```python
from build123d import *

# Parameters (mm, degrees)
F0_R     = 4.5
F0_W     = 85
F0_H     = 160
F0_H_2   = 10
F0_R_2   = 2
F1_DEPTH = 30
F2_W     = 85
F2_H     = 40
F2_R     = 4.5
F2_H_2   = 5
F3_DEPTH = 5
F4_W     = 85
F4_H     = 45
F4_R     = 2
F4_R_2   = 6
F5_DEPTH = 15
F4_R_3   = 4.5
F6_DEPTH = 15
F7_DEPTH = 25


with BuildPart() as f1:
    # F0 (on Top) → F1 (new body)
    with BuildSketch(Plane.XY):
        Polygon((115, -285), (115, 205), (265, 205), (265, 235), (-180, 235), (-180, 205), (-30, 205), (-30, -285), (-180, -285), (-180, -315), (265, -315), (265, -285), align=None)
        with Locations((-165, -300)):
            Circle(F0_R, mode=Mode.SUBTRACT)
        with Locations((250, -300)):
            Circle(F0_R, mode=Mode.SUBTRACT)
        Polygon((0, -120), (0, 0), (85, 0), (85, -120), (85, -130), (85, -285), (0, -285), (0, -130), align=None, mode=Mode.SUBTRACT)
        with Locations((27.5, 10)):
            Circle(F0_R, mode=Mode.SUBTRACT)
        with Locations((27.5, 29)):
            Circle(F0_R, mode=Mode.SUBTRACT)
        with Locations((-165, 220)):
            Circle(F0_R, mode=Mode.SUBTRACT)
        with Locations((57.5, 10)):
            Circle(F0_R, mode=Mode.SUBTRACT)
        with Locations((57.5, 29)):
            Circle(F0_R, mode=Mode.SUBTRACT)
        with Locations((42.5, 125)):
            Rectangle(F0_W, F0_H, mode=Mode.SUBTRACT)
        with Locations((250, 220)):
            Circle(F0_R, mode=Mode.SUBTRACT)
        with Locations((42.5, -125)):
            Rectangle(F0_W, F0_H_2)
        with Locations((10, -125)):
            Circle(F0_R_2, mode=Mode.SUBTRACT)
        with Locations((75, -125)):
            Circle(F0_R_2, mode=Mode.SUBTRACT)
    extrude(amount=F1_DEPTH)

    # F2 (on face) → F3 (cut)
    with BuildSketch(Plane.XY.offset(30)):
        with Locations((42.5, 20)):
            Rectangle(F2_W, F2_H)
        with Locations((27.5, 10)):
            Circle(F2_R, mode=Mode.SUBTRACT)
        with Locations((27.5, 29)):
            Circle(F2_R, mode=Mode.SUBTRACT)
        with Locations((57.5, 10)):
            Circle(F2_R, mode=Mode.SUBTRACT)
        with Locations((57.5, 29)):
            Circle(F2_R, mode=Mode.SUBTRACT)
        with Locations((42.5, 42.5)):
            Rectangle(F2_W, F2_H_2)
    extrude(amount=-F3_DEPTH, mode=Mode.SUBTRACT)

    # F4 (on face) + F0 (on Top) → F5 (cut)
    with BuildSketch(Plane.XY):
        with Locations((42.5, 22.5)):
            Rectangle(F4_W, F4_H)
        with Locations((10, 5)):
            Circle(F4_R, mode=Mode.SUBTRACT)
        with Locations((27.5, 10)):
            Circle(F4_R_2, mode=Mode.SUBTRACT)
        with Locations((10, 40)):
            Circle(F4_R, mode=Mode.SUBTRACT)
        with Locations((27.5, 29)):
            Circle(F4_R_2, mode=Mode.SUBTRACT)
        with Locations((57.5, 10)):
            Circle(F4_R_2, mode=Mode.SUBTRACT)
        with Locations((75, 5)):
            Circle(F4_R, mode=Mode.SUBTRACT)
        with Locations((57.5, 29)):
            Circle(F4_R_2, mode=Mode.SUBTRACT)
        with Locations((75, 40)):
            Circle(F4_R, mode=Mode.SUBTRACT)
    with BuildSketch(Plane.XY):
        with Locations((42.5, -125)):
            Rectangle(F0_W, F0_H_2)
        with Locations((10, -125)):
            Circle(F0_R_2, mode=Mode.SUBTRACT)
        with Locations((75, -125)):
            Circle(F0_R_2, mode=Mode.SUBTRACT)
    extrude(amount=F5_DEPTH, mode=Mode.SUBTRACT)

    # F4 (on face) → F6 (cut)
    with BuildSketch(Plane.XY):
        with Locations((27.5, 10)):
            Circle(F4_R_2)
        with Locations((27.5, 10)):
            Circle(F4_R_3, mode=Mode.SUBTRACT)
        with Locations((57.5, 10)):
            Circle(F4_R_2)
        with Locations((57.5, 10)):
            Circle(F4_R_3, mode=Mode.SUBTRACT)
        with Locations((57.5, 29)):
            Circle(F4_R_2)
        with Locations((57.5, 29)):
            Circle(F4_R_3, mode=Mode.SUBTRACT)
        with Locations((27.5, 29)):
            Circle(F4_R_2)
        with Locations((27.5, 29)):
            Circle(F4_R_3, mode=Mode.SUBTRACT)
    extrude(amount=F6_DEPTH, mode=Mode.SUBTRACT)

    # F4 (on face) → F7 (cut)
    with BuildSketch(Plane.XY):
        with Locations((10, 5)):
            Circle(F4_R)
        with Locations((10, 40)):
            Circle(F4_R)
        with Locations((75, 40)):
            Circle(F4_R)
        with Locations((75, 5)):
            Circle(F4_R)
    extrude(amount=F7_DEPTH, mode=Mode.SUBTRACT)


solid = f1.part
```
Check sheet for the modelled part. Datum: model origin and axes. Units: mm. A direction names the side the tool comes from. Coordinates: 2 decimals unless noted, no trailing zeros. Write each loop counter-clockwise with the first axis right and the second up, starting at its lowest first coordinate (ties: lowest second). Pieces come first, ordered by that corner, then holes. Notation, with made-up numbers: M -27.5,54 L -14.5,54 A11 ccw -14.5,62 Z; hole C -24.75,61 d2. An arc over 180 degrees is marked long. Write item = value, one per line. Start each with the question number.
1. Sectioned sample at B-B (x = 42.5). Record the cut outline in (y, z).
2. Go/stop test with flat-tipped pins: pin 1 (1 mm diameter, centred on y = -111, z = 22.5, fed in from +X); pin 2 (10 mm diameter, centred on y = 116, z = 12.5, fed in from -X); pin 3 (4.5 mm diameter, centred on x = 75, y = -125, fed in from -Z). Record where each tip stops, or that it passes through.
3. Thickness scan on probe 1 along Y at (x, z) = (-165, 19); probe 2 along Y at (x, z) = (1, 13.5); probe 3 along X at (y, z) = (-217, 28.25). Record the ranges inside material, lowest first.
4. Sectioned sample at A-A (y = -234). Record the cut outline in (x, z), then the cut area to 3 significant figures.
5. Sectioned sample at D-D (z = 8.5). Record the cut outline in (x, y).
6. Mould release check, pull along Y, two halves, no side actions. Record for faces 1 (the flat face through (265, -300, 15)), 2 (the flat face through (0, -43, 15)), 3 (the flat face through (39, -315, 15)): pulls with the +Y half, pulls with the -Y half, needs draft (parallel to the pull), parting line crosses it, or undercut.
7. Tool access check on faces 4 (the flat face through (42, 23, 25)), 5 (the flat face through (42, -120, 22)), 6 (the flat face through (-106, 205, 15)), 7 (the flat face through (115, -43, 15)). Record the directions out of +Z, -Z, +X, -X, +Y, -Y that give a thin tool (end or side, any length) a straight path to the whole face; none if there is none.
8. Sectioned sample at C-C (x = 235). Record the cut outline in (y, z).
The answers:
q1.outline = M -315,0 L -285,0 L -285,30 L -315,30 Z; M -130,15 L -120,15 L -120,30 L -130,30 Z; M 0,15 L 45,15 L 45,25 L 0,25 Z; M 205,0 L 235,0 L 235,30 L 205,30 Z
q2.pin_1 = 115
q2.pin_2 = -30
q2.pin_3 = 15
q3.probe_1 = -315 to -304.5, -295.5 to -285, 205 to 215.5, 224.5 to 235
q3.probe_2 = -315 to -285, 205 to 235
q3.probe_3 = -30 to 0, 85 to 115
q4.outline = M -30,0 L 0,0 L 0,30 L -30,30 Z; M 85,0 L 115,0 L 115,30 L 85,30 Z
q4.area = 1,800 mm²
q5.outline = M -180,-315 L 265,-315 L 265,-285 L 115,-285 L 115,205 L 265,205 L 265,235 L -180,235 L -180,205 L -30,205 L -30,-285 L -180,-285 Z; hole C -165,-300 d9; hole C -165,220 d9; hole M 0,-285 L 85,-285 L 85,205 L 0,205 Z; hole C 250,-300 d9; hole C 250,220 d9
q6.face_1 = needs draft
q6.face_2 = undercut
q6.face_3 = pulls with the -Y half
q7.face_4 = +Z
q7.face_5 = +Z, -Z
q7.face_6 = +Z, -Z, -X
q7.face_7 = +Z, -Z, +X
q8.outline = M -315,0 L -285,0 L -285,30 L -315,30 Z; M 205,0 L 235,0 L 235,30 L 205,30 Z
